Read the model definition and answer for the solid it produces. Units are mm, in the model's axes. A direction names the side the tool comes from. Give positions to 0.01 mm unless a question says otherwise; leave off trailing zeros. Write item = value, one per line.
```python
from build123d import *

# Parameters (mm, degrees)
SKETCH2_W          = 1282.7
SKETCH2_H          = 533.4
EXTRUDE1_DEPTH     = 17.78
SKETCH4_R          = 22.225
SKETCH4_R_2        = 1.5875
SKETCH4_R_3        = 1.628860789
SKETCH4_R_4        = 1.721410862
CUT_EXTRUDE1_DEPTH = 17.78
CUT_EXTRUDE2_DEPTH = 5.08


with BuildPart() as part:
    # Sketch2 → Extrude1 (new body)
    with BuildSketch(Plane.XY):
        with Locations((9556.220833334, -6075.3625)):
            Rectangle(SKETCH2_W, SKETCH2_H)
    extrude(amount=-EXTRUDE1_DEPTH)

    # Sketch4 → Cut-Extrude1 (cut)
    with BuildSketch(Plane.XY):
        with Locations((9051.395833334, -6281.7375)):
            Circle(SKETCH4_R)
        with Locations((9019.645833334, -6249.9875)):
            Circle(SKETCH4_R_2)
        with Locations((9083.145833334, -6249.9875)):
            Circle(SKETCH4_R_2)
        with Locations((9083.145833334, -6313.4875)):
            Circle(SKETCH4_R_3)
        with Locations((9019.645833334, -6313.4875)):
            Circle(SKETCH4_R_4)
        with Locations((9341.1675, -6265.8625)):
            Circle(SKETCH4_R_2)
        with Locations((9341.1675, -6138.8625)):
            Circle(SKETCH4_R_2)
        with Locations((9341.1675, -6011.8625)):
            Circle(SKETCH4_R_2)
        with Locations((9341.1675, -5884.8625)):
            Circle(SKETCH4_R_2)
        with Locations((9771.274166666, -5884.8625)):
            Circle(SKETCH4_R_2)
        with Locations((9771.274166666, -6011.8625)):
            Circle(SKETCH4_R_2)
        with Locations((9771.274166666, -6138.8625)):
            Circle(SKETCH4_R_2)
        with Locations((9771.274166666, -6265.8625)):
            Circle(SKETCH4_R_2)
        with BuildLine():
            Line((9974.787433334, -6061.075), (9974.787433334, -6045.241805286))
            ThreePointArc((9974.787433334, -6045.241805286), (9972.570596663, -6041.216758148), (9967.983861906, -6040.938848899))
            ThreePointArc((9967.983861906, -6040.938848899), (9957.371664972, -6048.421731638), (9949.888782233, -6059.033928571))
            ThreePointArc((9949.888782233, -6059.033928571), (9950.166691482, -6063.620663329), (9954.19173862, -6065.8375))
            Line((9954.19173862, -6065.8375), (9970.024933334, -6065.8375))
            ThreePointArc((9970.024933334, -6065.8375), (9973.39252938, -6064.442596045), (9974.787433334, -6061.075))
        make_face()
        with BuildLine():
            Line((9993.837433334, -6045.241805286), (9993.837433334, -6061.075))
            ThreePointArc((9993.837433334, -6061.075), (9995.232337289, -6064.442596045), (9998.599933334, -6065.8375))
            Line((9998.599933334, -6065.8375), (10014.433128046, -6065.8375))
            ThreePointArc((10014.433128046, -6065.8375), (10018.458175184, -6063.620663329), (10018.736084433, -6059.033928571))
            ThreePointArc((10018.736084433, -6059.033928571), (10011.253201696, -6048.421731637), (10000.641004763, -6040.938848899))
            ThreePointArc((10000.641004763, -6040.938848899), (9996.054270005, -6041.216758148), (9993.837433334, -6045.241805286))
        make_face()
        with BuildLine():
            Line((10014.433128046, -6084.8875), (9998.599933334, -6084.8875))
            ThreePointArc((9998.599933334, -6084.8875), (9995.232337289, -6086.282403955), (9993.837433334, -6089.65))
            Line((9993.837433334, -6089.65), (9993.837433334, -6105.483194714))
            ThreePointArc((9993.837433334, -6105.483194714), (9996.054270005, -6109.508241852), (10000.641004763, -6109.786151102))
            ThreePointArc((10000.641004763, -6109.786151102), (10011.253201699, -6102.303268365), (10018.736084435, -6091.691071429))
            ThreePointArc((10018.736084435, -6091.691071429), (10018.458175184, -6087.104336671), (10014.433128046, -6084.8875))
        make_face()
        with BuildLine():
            Line((9970.024933334, -6084.8875), (9954.19173862, -6084.8875))
            ThreePointArc((9954.19173862, -6084.8875), (9950.166691482, -6087.104336671), (9949.888782233, -6091.691071429))
            ThreePointArc((9949.888782233, -6091.691071429), (9957.371664972, -6102.303268362), (9967.983861906, -6109.786151101))
            ThreePointArc((9967.983861906, -6109.786151101), (9972.570596663, -6109.508241852), (9974.787433334, -6105.483194714))
            Line((9974.787433334, -6105.483194714), (9974.787433334, -6089.65))
            ThreePointArc((9974.787433334, -6089.65), (9973.39252938, -6086.282403955), (9970.024933334, -6084.8875))
        make_face()
        with BuildLine():
            ThreePointArc((9890.650044519, -6058.044318182), (9916.960512426, -6008.010579092), (9966.994251516, -5981.700111185))
            ThreePointArc((9966.994251516, -5981.700111185), (9972.584359078, -5978.426082773), (9974.787433334, -5972.333872304))
            ThreePointArc((9974.787433334, -5972.333872304), (9971.354643804, -5965.01194656), (9963.530615152, -5962.967633422))
            ThreePointArc((9963.530615152, -5962.967633422), (9903.490128244, -5994.54019491), (9871.917566756, -6054.580681818))
            ThreePointArc((9871.917566756, -6054.580681818), (9879.551987456, -6065.678738882), (9890.650044519, -6058.044318182))
        make_face()
        with BuildLine():
            ThreePointArc((9890.650044519, -6092.680681818), (9916.960512426, -6142.714420908), (9966.994251516, -6169.024888814))
            ThreePointArc((9966.994251516, -6169.024888814), (9974.628672216, -6180.122945878), (9963.530615152, -6187.757366578))
            ThreePointArc((9963.530615152, -6187.757366578), (9903.490128244, -6156.18480509), (9871.917566756, -6096.144318182))
            ThreePointArc((9871.917566756, -6096.144318182), (9879.551987456, -6085.046261119), (9890.650044519, -6092.680681818))
        make_face()
        with BuildLine():
            ThreePointArc((10001.630615152, -6169.024888815), (10051.664354242, -6142.714420908), (10077.974822149, -6092.680681818))
            ThreePointArc((10077.974822149, -6092.680681818), (10089.072879212, -6085.046261118), (10096.707299912, -6096.144318182))
            ThreePointArc((10096.707299912, -6096.144318182), (10065.134738424, -6156.18480509), (10005.094251516, -6187.757366578))
            ThreePointArc((10005.094251516, -6187.757366578), (9993.996194453, -6180.122945878), (10001.630615152, -6169.024888815))
        make_face()
        with BuildLine():
            ThreePointArc((10001.630615152, -5981.700111185), (10051.664354242, -6008.010579092), (10077.974822148, -6058.044318182))
            ThreePointArc((10077.974822148, -6058.044318182), (10089.072879212, -6065.678738882), (10096.707299912, -6054.580681818))
            ThreePointArc((10096.707299912, -6054.580681818), (10065.134738424, -5994.54019491), (10005.094251516, -5962.967633422))
            ThreePointArc((10005.094251516, -5962.967633422), (9993.996194453, -5970.602054122), (10001.630615152, -5981.700111185))
        make_face()
        with BuildLine():
            ThreePointArc((9917.282231904, -6111.603251872), (9908.112433335, -6075.3625), (9917.282231902, -6039.121748127))
            ThreePointArc((9917.282231902, -6039.121748127), (9930.191101067, -6035.273066932), (9934.039782262, -6048.181936096))
            ThreePointArc((9934.039782262, -6048.181936096), (9927.162433334, -6075.3625), (9934.039782262, -6102.543063904))
            ThreePointArc((9934.039782262, -6102.543063904), (9930.191101067, -6115.451933067), (9917.282231904, -6111.603251872))
        make_face()
        with BuildLine():
            ThreePointArc((9948.071681461, -6008.332298571), (9984.312433334, -5999.162500001), (10020.553185206, -6008.33229857))
            ThreePointArc((10020.553185206, -6008.33229857), (10024.401866401, -6021.241167734), (10011.492997237, -6025.089848928))
            ThreePointArc((10011.492997237, -6025.089848928), (9984.312433332, -6018.212500002), (9957.131869429, -6025.089848928))
            ThreePointArc((9957.131869429, -6025.089848928), (9944.223000266, -6021.241167734), (9948.071681461, -6008.332298571))
        make_face()
        with BuildLine():
            ThreePointArc((10020.553185206, -6142.39270143), (9984.312433334, -6151.5625), (9948.071681462, -6142.39270143))
            ThreePointArc((9948.071681462, -6142.39270143), (9944.223000267, -6129.483832267), (9957.13186943, -6125.635151072))
            ThreePointArc((9957.13186943, -6125.635151072), (9984.312433334, -6132.5125), (10011.492997238, -6125.635151072))
            ThreePointArc((10011.492997238, -6125.635151072), (10024.401866401, -6129.483832267), (10020.553185206, -6142.39270143))
        make_face()
        with BuildLine():
            ThreePointArc((10051.342634764, -6039.121748128), (10060.512433334, -6075.362500001), (10051.342634763, -6111.603251873))
            ThreePointArc((10051.342634763, -6111.603251873), (10038.43373034, -6115.45201683), (10034.585084407, -6102.543063904))
            ThreePointArc((10034.585084407, -6102.543063904), (10041.481307607, -6075.344363194), (10034.638226606, -6048.13224352))
            ThreePointArc((10034.638226606, -6048.13224352), (10038.489557591, -6035.282901746), (10051.342634764, -6039.121748128))
        make_face()
    extrude(amount=-CUT_EXTRUDE1_DEPTH, mode=Mode.SUBTRACT)

    # Sketch5 → Cut-Extrude2 (cut)
    with BuildSketch(Plane.XY):
        Polygon((9350.0575, -6075.3625), (9350.0575, -5808.6625), (9332.2775, -5808.6625), (9332.2775, -6342.0625), (9350.0575, -6342.0625), align=None)
        Polygon((9762.384166666, -6075.3625), (9762.384166666, -6342.0625), (9780.164166666, -6342.0625), (9780.164166666, -5808.6625), (9762.384166666, -5808.6625), align=None)
    extrude(amount=-CUT_EXTRUDE2_DEPTH, mode=Mode.SUBTRACT)


solid = part.part
```
1) Find the intervals of material crossed by probe 1 along X at (y, z) = (-6234.5, -4.75); probe 2 along X at (y, z) = (-6269.5, -2.75); probe 3 along X at (y, z) = (-5998.5, -4), in increasing order.
Output:
probe_1 = 8914.87 to 9332.28, 9350.06 to 9762.38, 9780.16 to 10197.57
probe_2 = 8914.87 to 9032.84, 9069.95 to 9332.28, 9350.06 to 9762.38, 9780.16 to 10197.57
probe_3 = 8914.87 to 9332.28, 9350.06 to 9762.38, 9780.16 to 9899.72, 9928.06 to 10040.57, 10068.91 to 10197.57
2) This flat-tipped pin is pushed along its axis until it touches: P1, Ø3.5, axis at x = 9771.27, y = -6138.86, coming from the +Z side. Where does it stop, or does it pass through?
Output:
P1 = -5.08
3) The mould has two halves that part along X. Classify faces 1 (the face through (9547, -6072, -17.78)), 2 (the face through (9046.578, -6303.434, -8.766)): pulls with the +X half, pulls with the -X half, needs draft (parallel to the pull), parting line crosses it, or undercut.
Output:
face_1 = needs draft
face_2 = undercut
4) A cutting plane is placed at A-A on z = -11.5. Give the number of separate pieces and of enclosed holes in the cut face, then the cut area to 3 significant figures.
Output:
separate_pieces = 1
enclosed_holes = 25
area = 664,000 mm²
5) A tool of negligible diameter and unlimited length cuts with its end or side. For faces 3 (the face through (10065.81, -5995.22, -8.77)), 4 (the face through (9986, -6072, 0)), from which of +Z, -Z, +X, -X, +Y, -Y can it reach the whole face along a straight path? Write none if from no direction.
Output:
face_3 = +Z, -Z
face_4 = +Z, +X, -X, +Y, -Y
